Could you check a few things on this model? Use its own coordinates, in mm. Face numbers are marked on the shaded views. A direction names the side the tool comes from. Coordinates: 2 decimals unless noted, no trailing zeros. Write each loop counter-clockwise with the first axis right and the second up, starting at its lowest first coordinate (ties: lowest second). Pieces come first, ordered by that corner, then holes. Notation, with made-up numbers: (52.25, -21.75) - (101.25, -21.75) arc R20 cw to (101.25, -6.75) - close; hole circle Ø8 at (-38.75, 22.5). An arc over 180 degrees is marked (long way). Write item = value, one per line. Start each with the question number.
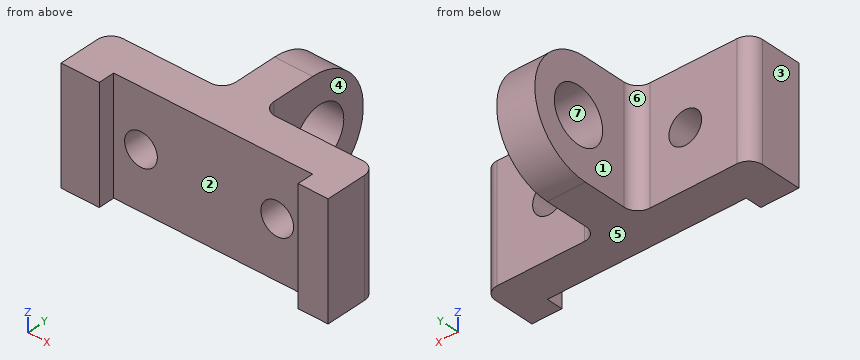
```python
from build123d import *

# Parameters (mm, degrees)
SKETCH1_W                = 98
SKETCH1_H                = 42
BOSS_EXTRUDE1_DEPTH      = 14
BOSS_EXTRUDE2_DEPTH      = 21
BOSS_EXTRUDE2_DEPTH_BACK = 21
SKETCH2_W                = 11.017552575
SKETCH2_H                = 6
FILLET1_R                = 5
SKETCH3_W                = 14
SKETCH3_H                = 6
BOSS_EXTRUDE3_DEPTH      = 42
FILLET2_R                = 5
SKETCH4_R                = 6
CUT_EXTRUDE1_DEPTH       = 14
BOSS_EXTRUDE4_DEPTH      = 7
BOSS_EXTRUDE4_DEPTH_BACK = 7
SKETCH5_R                = 10
FILLET3_R                = 5
FILLET4_R                = 5


with BuildPart() as part:
    # Sketch1 → Boss-Extrude1 (new body)
    with BuildSketch(Plane(origin=(0, 0, 0), x_dir=(1, 0, 0), z_dir=(0, 1, 0))):
        Rectangle(SKETCH1_W, SKETCH1_H)
    extrude(amount=BOSS_EXTRUDE1_DEPTH)

    # Sketch2 → Boss-Extrude2 (add, two sides: drawn at the far end of the back side and taken through both)
    with BuildSketch(Plane.XY.offset(-BOSS_EXTRUDE2_DEPTH_BACK)):
        with Locations((43.491223713, -3)):
            Rectangle(SKETCH2_W, SKETCH2_H)
    extrude(amount=BOSS_EXTRUDE2_DEPTH + BOSS_EXTRUDE2_DEPTH_BACK)

    # Fillet1
    fillet1_edges = [part.edges().sort_by_distance(p)[0] for p in [
        (49, 14, 0),
    ]]
    fillet(fillet1_edges, radius=FILLET1_R)

    # Sketch3 → Boss-Extrude3 (add)
    with BuildSketch(Plane.XY.offset(21)):
        with Locations((-42, -3)):
            Rectangle(SKETCH3_W, SKETCH3_H)
    extrude(amount=-BOSS_EXTRUDE3_DEPTH)

    # Fillet2
    fillet2_edges = [part.edges().sort_by_distance(p)[0] for p in [
        (-49, 14, 0),
    ]]
    fillet(fillet2_edges, radius=FILLET2_R)

    # Sketch4 → Cut-Extrude1 (cut)
    with BuildSketch(Plane(origin=(0, 0, 0), x_dir=(1, 0, 0), z_dir=(0, 1, 0))):
        with Locations(Location((25, 0, 0), (0, 0, 270))):
            Circle(SKETCH4_R)
        with Locations(Location((-25, 0, 0), (0, 0, 90))):
            Circle(SKETCH4_R)
    extrude(amount=CUT_EXTRUDE1_DEPTH, mode=Mode.SUBTRACT)

    # Sketch5 → Boss-Extrude4 (add, two sides: drawn at the far end of the back side and taken through both)
    with BuildSketch(Plane(origin=(0, 0, 0), x_dir=(0, 0, -1), z_dir=(1, 0, 0)).offset(-BOSS_EXTRUDE4_DEPTH_BACK)):
        with BuildLine():
            Line((-21, 14), (-21, 35))
            ThreePointArc((-21, 35), (0, 56), (21, 35))
            Line((21, 35), (21, 14))
            Line((21, 14), (-21, 14))
        make_face()
        with Locations((0, 37.895751368)):
            Circle(SKETCH5_R, mode=Mode.SUBTRACT)
    extrude(amount=BOSS_EXTRUDE4_DEPTH + BOSS_EXTRUDE4_DEPTH_BACK)

    # Fillet3
    fillet3_edges = [part.edges().sort_by_distance(p)[0] for p in [
        (7, 14, 0),
    ]]
    fillet(fillet3_edges, radius=FILLET3_R)

    # Fillet4
    fillet4_edges = [part.edges().sort_by_distance(p)[0] for p in [
        (-7, 14, 0),
    ]]
    fillet(fillet4_edges, radius=FILLET4_R)


solid = part.part
```
1) Suppose I cut it at A-A on x = -25. Please give me the cut outline in (y, z), plus the area to 3 significant figures.
2) For P1, Ø9.5, axis at x = -25, z = 0, coming from the -Y side; P2, Ø14, axis at x = 25, z = 0, coming from the +Y side; P3, Ø2, axis at y = 11, z = -7.5, coming from the +X side; P4, Ø11, axis at y = 42, z = -10, coming from the -X side, each with a flat end and sliding along its axis, tell me the tip position at first contact or that it passes through.
3) Which directions (+Z, -Z, +X, -X, +Y, -Y) give clear straight access to the entire face, cutting with the end or side of a thin tool? Please do the marked faces 1, 2, 3 and 4.
4) Suppose I cut it at C-C on z = -4. Please give me the cut outline in (x, y).
5) Suppose I cut it at B-B on y = 43. Please give me the cut outline in (x, z), plus the area to 3 significant figures.
6) If I drill on probe 1 along X at (y, z) = (3.5, 0); probe 2 along Y at (x, z) = (4.25, 0); probe 3 along Z at (x, y) = (-25, 4.75), over which ranges is the centre line in solid material (lowest first)? Write a range as [from, to].
7) Thinking about a two-plate mould opening in Y: for the marked faces 5, 6 and 7, which applies, +Y half, -Y half, draft (parallel to the pull), parting line (faces both ways), or undercut?
8) Suppose I cut it at D-D on y = 6.5. Please give me the cut outline in (x, z).
Reply:
q1.outline = (0, -21) - (14, -21) - (14, -6) - (0, -6) - close; (0, 6) - (14, 6) - (14, 21) - (0, 21) - close
q1.area = 420 mm^2
q2.P1 = through
q2.P2 = 14
q2.P3 = 48.9
q2.P4 = -7
q3.face_1 = +Z, -Z, -X, +Y
q3.face_2 = +Z, -Z, -Y
q3.face_3 = +Z, -Z, -X, +Y, -Y
q3.face_4 = +Z, -Z, +X, +Y
q4.outline = (-49, -6) - (-35, -6) - (-35, 0) - (-29.47, 0) - (-29.47, 14) - (-44, 14) arc R5 ccw to (-49, 9) - close; (-20.53, 0) - (20.53, 0) - (20.53, 14) - (12, 14) arc R5 cw to (7, 19) - (7, 28.73) - (-7, 28.73) - (-7, 19) arc R5 cw to (-12, 14) - (-20.53, 14) - close; (-7, 47.06) - (7, 47.06) - (7, 55.62) - (-7, 55.62) - close; (29.47, 0) - (37.98, 0) - (37.98, -6) - (49, -6) - (49, 9) arc R5 ccw to (44, 14) - (29.47, 14) - close
q5.outline = (-7, -19.42) - (7, -19.42) - (7, -8.6) - (-7, -8.6) - close; (-7, 8.6) - (7, 8.6) - (7, 19.42) - (-7, 19.42) - close
q5.area = 303 mm^2
q6.probe_1 = [-49, -31], [-19, 19], [31, 49]
q6.probe_2 = [0, 27.9], [47.9, 56]
q6.probe_3 = [-21, -6], [6, 21]
q7.face_5 = draft
q7.face_6 = +Y half
q7.face_7 = undercut
q8.outline = (-49, -21) - (49, -21) - (49, 21) - (-49, 21) - close; hole circle Ø12 at (-25, 0); hole circle Ø12 at (25, 0)
